Verification items for the finished model (mm, model axes). A direction names the side the tool comes from. Coordinates: 2 decimals unless noted, no trailing zeros. Loops run counter-clockwise (first coordinate to the right, second up) from the corner with the lowest first, then second, coordinate; pieces in that order, holes last.
Q1. Sectioned sample at D-D (z = 0). Enter the section's corners in (x, y).
Q2. Go/stop test with flat-tipped pins: P1, Ø2, axis at x = -6.5, z = 0.5, coming from the +Y side; P2, Ø0.9, axis at y = 2.5, z = 1, coming from the +X side; P3, Ø1, axis at x = -11.5, z = -0.5, coming from the +Y side. Record where each tip stops, or that it passes through.
Q3. Mould release check, pull along Z, two halves, no side actions. Record for faces 3 (the face through (-17.678, 1.805, 1.311)), 4 (the face through (-18, 2, 3)), 5 (the face through (0, 2, 1)): +Z half, -Z half, draft (parallel to the pull), parting line (faces both ways), or undercut.
Q4. Sectioned sample at A-A (x = -20). Enter the section's corners in (y, z), then the cut area to 3 significant figures.
Q5. Sectioned sample at C-C (y = 1.15). Enter the section's corners in (x, z), then the cut area to 3 significant figures.
Q6. Material ranges on probe 1 along X at (y, z) = (2.15, 0.2); probe 2 along Z at (x, y) = (-10.5, 2.55); probe 3 along Z at (x, y) = (-8, 1.55), recorded low to high.
Q7. Access from +Z, -Z, +X, -X, +Y, -Y to the whole of each face (thin tool, end or side, straight path). Record for faces 1 (the face through (-18, 0, 0)), 2 (the face through (-4.8, 2, 1)).
Q8. Sectioned sample at B-B (z = 1.3). Enter the section's corners in (x, y), then the cut area to 3 significant figures.
```python
from build123d import *

# Parameters (mm, degrees)
TOP_SKETCH_W                 = 35
TOP_SKETCH_H                 = 5
THICKNESS_EXTRUDE_DEPTH      = 3.5
HANDLE_SKETCH_W              = 25.4
HANDLE_SKETCH_H              = 3.2
HANDLE_SLOT_CUT_DEPTH        = 3.1
HANDLE_SLOT_CHAMFER_1_SIZE   = 1.6
HANDLE_SLOT_CHAMFER_1_SIZE2  = 2.771281292
HANDLE_SLOT_CHAMFER_2_SIZE   = 1.6
HANDLE_SLOT_CHAMFER_2_SIZE_2 = 2.771281292


with BuildPart() as part:
    # Top Sketch → Thickness Extrude (new body)
    with BuildSketch(Plane(origin=(0, 0, 0), x_dir=(1, 0, 0), z_dir=(0, 1, 0))):
        with Locations((-17.5, -0.5)):
            Rectangle(TOP_SKETCH_W, TOP_SKETCH_H)
    extrude(amount=THICKNESS_EXTRUDE_DEPTH)

    # Handle Sketch → Handle Slot Cut (cut)
    with BuildSketch(Plane(origin=(0, 3.5, 0), x_dir=(1, 0, 0), z_dir=(0, 1, 0))):
        with Locations((-17.5, -0.5)):
            Rectangle(HANDLE_SKETCH_W, HANDLE_SKETCH_H)
    extrude(amount=-HANDLE_SLOT_CUT_DEPTH, mode=Mode.SUBTRACT)

    # Handle Slot Chamfer 1
    handle_slot_chamfer_1_edges = [part.edges().sort_by_distance(p)[0] for p in [
        (-17.5, 0.4, 2.1),
    ]]
    handle_slot_chamfer_1_side = [part.faces().sort_by_distance(p)[0] for p in [
        (-17.5, 0.4, 0.5),
    ]]
    chamfer(handle_slot_chamfer_1_edges, length=HANDLE_SLOT_CHAMFER_1_SIZE, length2=HANDLE_SLOT_CHAMFER_1_SIZE2, reference=handle_slot_chamfer_1_side[0])

    # Handle Slot Chamfer 2
    # the kernel refuses this chamfer: 2.771281292, 1.6 mm, written as the material it adds along each edge
    with BuildSketch(Plane(origin=(-37.369542353, 0.4, -1.1), x_dir=(0, -0.057893862402671414, 0.9983227437537925), z_dir=(1, 0, 0))) as handle_slot_chamfer_2_piece_1_section:
        Polygon((HANDLE_SLOT_CHAMFER_2_SIZE * 0.998322743754, -HANDLE_SLOT_CHAMFER_2_SIZE * 0.0578938624027), (-HANDLE_SLOT_CHAMFER_2_SIZE_2 * 0.057893862405, -HANDLE_SLOT_CHAMFER_2_SIZE_2 * 0.998322743793), (0, 0), align=None)
    handle_slot_chamfer_2_piece_1 = extrude(amount=39.739084706, mode=Mode.PRIVATE)
    handle_slot_chamfer_2_piece_1 = split(handle_slot_chamfer_2_piece_1, bisect_by=Plane(origin=(-35, 1.323760431, -0.566666667), z_dir=(1, 0, 0)), keep=Keep.TOP, mode=Mode.PRIVATE)
    handle_slot_chamfer_2_piece_1 = split(handle_slot_chamfer_2_piece_1, bisect_by=Plane(origin=(0, 1.323760431, -0.566666667), z_dir=(-1, 0, 0)), keep=Keep.TOP, mode=Mode.PRIVATE)
    add(handle_slot_chamfer_2_piece_1)


solid = part.part
```
Geometry check:
1. outline: (-35, 0) - (0, 0) - (0, 3.5) - (-4.8, 3.5) - (-4.8, 1.27) - (-30.2, 1.27) - (-30.2, 3.5) - (-35, 3.5) - close
2. P1: stops at y = 2.13
2. P2: stops at x = 0
2. P3: stops at y = 3
3. face 3: undercut
3. face 4: +Z half
3. face 5: draft
4. outline: (0, -2) - (3.5, -2) - (3.5, -1.1) - (3.17, -1.1) - (0.4, 0.5) - (3.17, 2.1) - (3.5, 2.1) - (3.5, 3) - (0, 3) - close
4. area: 12.0 mm2
5. outline: (-35, -2) - (0, -2) - (0, 3) - (-35, 3) - close; hole (-30.2, 0.07) - (-4.8, 0.07) - (-4.8, 0.93) - (-30.2, 0.93) - close
5. area: 153 mm2
6. probe 1: x = -35 to -30.2, -4.8 to 0
6. probe 2: z = -2 to -0.74, 1.74 to 3
6. probe 3: z = -2 to -0.16, 1.16 to 3
7. face 1: +Z, -Z, +X, -X, -Y
7. face 2: +Y
8. outline: (-35, 0) - (0, 0) - (0, 3.5) - (-4.8, 3.5) - (-4.8, 1.79) - (-30.2, 1.79) - (-30.2, 3.5) - (-35, 3.5) - close
8. area: 79.0 mm2
